Solid Edge part; units mm, degrees
sketch "Sketch1" plane through (0, 0, 0) normal (0, -1, 0) x (1, 0, 0)
  line L0 (-6, 8) -> (6, 8)
  line L1 (6, 8) -> (6, 0)
  line L2 (6, 0) -> (-6, 0)
  line L3 (-6, 0) -> (-6, 8)
  dimension "D1" = 6
  dimension "D2" = 6
extrude "Protrusion1" add sketch "Sketch1" along normal mid plane 370
sketch "Sketch2" plane through (0, 0, 8) normal (0, 0, 1) x (0, 1, 0)
  circle A0 centre (175, 0) radius 1.75
extrude "Cutout1" cut sketch "Sketch2" against normal through all
sketch "Sketch3" plane through (0, 0, 8) normal (0, 0, 1) x (0, 1, 0)
  circle A0 centre (175, 0) radius 3
extrude "ExtrudedCutout_2" cut sketch "Sketch3" against normal blind 4.5
pattern_linear "Pattern1" count 15 spacing 25 along (0, -1, 0) of "Cutout1", "ExtrudedCutout_2"
properties material "Stainless Steel, 410"
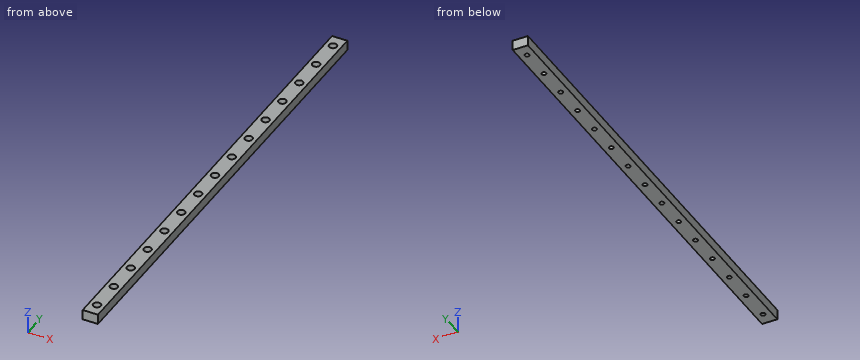
The model under review builds one solid part; all positions refer to its coordinate system, in mm. Give positions to 0.01 mm unless a question says otherwise; leave off trailing zeros. Put each result on its own line as item: value.
(1) To check wall thickness, follow probe 1 along X at (y, z) = (-125, 1.6); probe 2 along X at (y, z) = (-75, 7.15); probe 3 along Z at (x, y) = (2.75, -126). State the ranges of each line that lie inside material, in increasing order. Write a range as from..to.
Results are:
probe 1: -6..-1.75, 1.75..6
probe 2: -6..-3, 3..6
probe 3: 0..3.5
(2) We need section A-A, the plane z = 6.25. State how many separate pieces and enclosed holes the cut face has, and give its area (3 significant figures).
Results are:
separate pieces: 1
enclosed holes: 15
area: 4,020 mm²
(3) For pin 1 Ø4.5 at (x, y) = (0, 0) entering from +Z; pin 2 Ø3 at (x, y) = (0, -100) entering from +Z, all flat-tipped, find the tip position at first contact; note any pin that passes through.
Results are:
pin 1: z = 3.5
pin 2: through
